Source: CAD feature listing. Evaluate the final solid. Frame: model axes, mm. A direction names the side the tool comes from. Coordinates: 2 decimals unless noted, no trailing zeros. Write each loop counter-clockwise with the first axis right and the second up, starting at its lowest first coordinate (ties: lowest second). Pieces come first, ordered by that corner, then holes. Notation, with made-up numbers: M 75.25,-8 L 88.25,-8 A9 cw 88.25,-1 Z; hole C 70,-14.75 d1. An arc over 180 degrees is marked long. Write item = value, one per line. Start each with the question number.
1. Line query: line 1 along Y through (x, z) = (-9.75, 0); line 2 along Y through (x, z) = (0, 1.5); line 3 along Z through (x, y) = (-11.5, 7.5). Output: solid intervals per line, ascending.
2. Section query A-A (x = 0). Output: boundary loops of the cut face in (y, z), then the cut area to 3 significant figures.
3. Pull-direction query (Z, two-part tool) for faces 6 (the face through (4, 9, -4)), 7 (the face through (-5.29, 0.64, 5.01)), 8 (the face through (5.76, 7.93, 0.06)); classes: pulls with the +Z half, pulls with the -Z half, needs draft (parallel to the pull), parting line crosses it, or undercut.
4. Section query C-C (x = 9). Output: boundary loops of the cut face in (y, z), then the cut area to 3 significant figures.
5. Pin query (flat end, axial travel): pin 1 Ø8 at (x, y) = (-4.5, 13) entering from +Z; pin 2 Ø7.5 at (x, y) = (0, 10) entering from -Z; pin 3 Ø7.5 at (x, y) = (0.5, 4.5) entering from +Z; pin 4 Ø4.5 at (y, z) = (7.5, 0) entering from +X. Return the tip coordinate at first contact, or that it passes through.
6. Section query B-B (z = 3.25). Output: boundary loops of the cut face in (x, y), then the cut area to 3 significant figures.
7. Section query D-D (y = 12.75). Output: boundary loops of the cut face in (x, z).
8. Access query for faces 1 (the face through (-8, 7.4, -5)), 2 (the face through (-17, 7, -3)), 3 (the face through (5.29, 14.36, 5.01)), 4 (the face through (-11.93, 5.06, 0.54)), 5 (the face through (0, 15, 0)). Directions: +Z, -Z, +X, -X, +Y, -Y. A direction counts if a zero-diameter tool reaches every point of the face in a straight line with its end or side. Return the directions, or none.
```python
from build123d import *

# Parameters (mm, degrees)
SKETCH_1_W          = 34
SKETCH_1_H          = 12
EXTRUDE_1_DEPTH     = 15
SKETCH_2_R          = 4
CUT_EXTRUDE_1_DEPTH = 26.651510677
M6X1_0_2_D          = 5
M6X1_0_2_DEPTH      = 10
M6X1_0_2_TIP        = 1.502151548
M6X1_0_1_D          = 5
M6X1_0_1_DEPTH      = 10
M6X1_0_1_TIP        = 1.502151548
SKETCH_11_R         = 8
CUT_EXTRUDE_2_DEPTH = 2
CUT_EXTRUDE_START   = -2
SKETCH_12_R         = 8
CUT_EXTRUDE_3_DEPTH = 2
FILLET_1_R          = 1


with BuildPart() as part:
    # 草图1 → 凸台-拉伸1 (new body)
    with BuildSketch(Plane(origin=(0, 0, 0), x_dir=(1, 0, 0), z_dir=(0, 1, 0))):
        Rectangle(SKETCH_1_W, SKETCH_1_H)
    extrude(amount=EXTRUDE_1_DEPTH)

    # 草图2 → 切除-拉伸1 (cut, through all)
    with BuildSketch(Plane(origin=(0, 0, -6), x_dir=(-1, 0, 0), z_dir=(0, 0, -1))):
        with Locations((0, 7.5)):
            Circle(SKETCH_2_R)
    extrude(amount=-CUT_EXTRUDE_1_DEPTH, mode=Mode.SUBTRACT)

    # M6x1.0 螺纹孔2
    with Locations(Plane.ZY.offset(17)):
        with Locations((0, 7.5)):
            Hole(M6X1_0_2_D / 2, depth=M6X1_0_2_DEPTH)
            with Locations((0, 0, -(M6X1_0_2_DEPTH + M6X1_0_2_TIP / 2))):  # 118° drill point
                Cone(0, M6X1_0_2_D / 2, M6X1_0_2_TIP, mode=Mode.SUBTRACT)

    # M6x1.0 螺纹孔1
    with Locations(Plane(origin=(17, 0, 0), x_dir=(0, 0, -1), z_dir=(1, 0, 0))):
        with Locations((0, 7.5)):
            Hole(M6X1_0_1_D / 2, depth=M6X1_0_1_DEPTH)
            with Locations((0, 0, -(M6X1_0_1_DEPTH + M6X1_0_1_TIP / 2))):  # 118° drill point
                Cone(0, M6X1_0_1_D / 2, M6X1_0_1_TIP, mode=Mode.SUBTRACT)

    # 草图11 → 切除-拉伸2 (cut)
    with BuildSketch(Plane.XY.offset(6)):
        with Locations((0, 7.5)):
            Circle(SKETCH_11_R)
    extrude(amount=-CUT_EXTRUDE_2_DEPTH, mode=Mode.SUBTRACT)

    # 草图12 → 切除-拉伸3 (cut)
    with BuildSketch(Plane(origin=(0, 0, -6), x_dir=(-1, 0, 0), z_dir=(0, 0, -1)).offset(CUT_EXTRUDE_START)):
        with Locations((0, 7.5)):
            Circle(SKETCH_12_R)
    extrude(amount=CUT_EXTRUDE_3_DEPTH, mode=Mode.SUBTRACT)

    # 圆角1
    fillet_1_edges = [part.edges().sort_by_distance(p)[0] for p in [
        (2.783882181, 0, 5),
        (-2.783882181, 0, 5),
        (-2.783882181, 15, 5),
        (2.783882181, 15, 5),
        (-2.783882181, 0, -5),
        (2.783882181, 0, -5),
        (2.783882181, 15, -5),
        (-2.783882181, 15, -5),
    ]]
    fillet(fillet_1_edges, radius=FILLET_1_R)


solid = part.part
```
Results are:
q1.line_1 = 0 to 5, 10 to 15
q1.line_2 = 0 to 3.5, 11.5 to 15
q1.line_3 = -6 to -2.5, 2.5 to 6
q2.outline = M 0,-4 L 3.5,-4 L 3.5,4 L 0,4 Z; M 11.5,-4 L 15,-4 L 15,4 L 11.5,4 Z
q2.area = 56.0 mm^2
q3.face_6 = pulls with the -Z half
q3.face_7 = needs draft
q3.face_8 = undercut
q4.outline = M 0,-6 L 15,-6 L 15,6 L 0,6 Z; hole C 7.5,0 d5
q4.area = 160 mm^2
q5.pin_1 = 6
q5.pin_2 = -4
q5.pin_3 = 4
q5.pin_4 = 6.85
q6.outline = M -17,0 L 17,0 L 17,15 L -17,15 Z; hole C 0,7.5 d8
q6.area = 460 mm^2
q7.outline = M -17,-6 L -6.04,-6 L -6.04,-4 L 6.04,-4 L 6.04,-6 L 17,-6 L 17,6 L 6.04,6 L 6.04,4 L -6.04,4 L -6.04,6 L -17,6 Z
q8.face_1 = -Z
q8.face_2 = +Z, -Z, -X, +Y, -Y
q8.face_3 = +Z
q8.face_4 = -X
q8.face_5 = +Z, -Z, +X, -X, +Y
